Autodesk Inventor part; units mm, degrees
ref_plane "YZ Plane" through (0, 0, 0) normal (1, 0, 0) x (0, 1, 0)
ref_plane "XZ Plane" through (0, 0, 0) normal (0, 1, 0) x (-1, 0, 0)
ref_plane "XY Plane" through (0, 0, 0) normal (0, 0, 1) x (1, 0, 0)
sketch "Sketch1" plane through (0, 0, 0) normal (0, 0, 1) x (1, 0, 0)
  line L0 (-23, -40) -> (23, -40)
  line L1 (23, -40) -> (23, 40)
  line L2 (23, 40) -> (-23, 40)
  line L3 (-23, 40) -> (-23, -40)
  line L4 (-23, -40) -> (23, 40) construction
  line L5 (23, -40) -> (-23, 40) construction
  line L6 (10, -20) -> (-10, -20)
  line L7 (-10, -20) -> (-10, 20)
  line L8 (-10, 20) -> (10, 20)
  line L9 (10, 20) -> (10, -20)
  line L10 (10, -20) -> (-10, 20) construction
  line L11 (-10, -20) -> (10, 20) construction
  point P0 (0, 0)
  dimension "d154" = 46
  dimension "d155" = 80
  dimension "d172" = 20
  dimension "d181" = 40
extrude "Plate5" add sketch "Sketch1" along normal blind 3 contours L3 L2 L1 L0 | L6 L7 L8 L9
sketch "Sketch9" plane through (0, 0, 3) normal (0, 0, 1) x (1, 0, 0)
  circle A0 centre (16.7705, -33.541) radius 3
  line L0 (16.7705, 33.541) -> (-16.7705, 33.541) construction
  line L1 (-16.7705, 33.541) -> (-16.7705, -33.541) construction
  line L2 (-16.7705, -33.541) -> (16.7705, -33.541) construction
  line L3 (16.7705, -33.541) -> (16.7705, 33.541) construction
  line L4 (16.7705, 33.541) -> (-16.7705, -33.541) construction
  line L5 (-16.7705, 33.541) -> (16.7705, -33.541) construction
  circle A1 centre (-16.7705, -33.541) radius 3
  circle A2 centre (16.7705, 33.541) radius 3
  circle A3 centre (-16.7705, 33.541) radius 3
  circle A4 centre (0, 0) radius 37.5 construction
  line L6 (23, -40) -> (-23, -40) construction
  line L7 (23, 40) -> (23, -40) construction
  line L8 (-23, 40) -> (23, 40) construction
  line L9 (-23, -40) -> (-23, 40) construction
  circle A5 centre (0, 0) radius 22.3607 construction
  line L10 (10, 20) -> (-10, -20) construction
  dimension "d180" = 75
  dimension "d182" = 15.1393
  dimension "d174" = 6
  dimension "d183" = 33.541
extrude "Cut2" cut sketch "Sketch9" against normal blind 3
fillet "Corner Round1" radius 6 4 edges at (23, 40, 1.5) (-23, 40, 1.5) (-23, -40, 1.5) (23, -40, 1.5)
feature "Corner Round2" [suppressed]
properties part number "ANP 1434 BOTTOM FDS support flange" material "Stainless Steel"
The listing builds one solid part. Answer for the finished solid, in the listing's coordinates (mm). Coordinates: 2 decimals unless noted, no trailing zeros. Write each loop counter-clockwise with the first axis right and the second up, starting at its lowest first coordinate (ties: lowest second). Pieces come first, ordered by that corner, then holes.
Q1. Given P1, Ø5.5, axis at x = -16.77, y = 33.54, coming from the -Z side, flat-ended and moving along its own axis, determine where the tip first touches the part or whether it passes through.
Returned:
P1: passes through
Q2. The mould has two halves that part along Y. Classify faces 1 (the cylindrical face through (-21.289, -38.196, 1.521)), 2 (the cylindrical face through (-15.16, 36.07, 1.52)), 3 (the flat face through (23, 0, 1)), 4 (the cylindrical face through (-21.196, 38.289, 1.521)): released by +Y, released by -Y, zero draft, split by the parting line, or undercut.
Returned:
face 1: released by -Y
face 2: undercut
face 3: zero draft
face 4: released by +Y
Q3. Section A-A, the plane x = -15 is taken. Write down the section's boundary in (y, z), then the cut area to 3 significant figures.
Returned:
outline: (-40, 0) - (-35.96, 0) - (-35.96, 3) - (-40, 3) - close; (-31.12, 0) - (31.12, 0) - (31.12, 3) - (-31.12, 3) - close; (35.96, 0) - (40, 0) - (40, 3) - (35.96, 3) - close
area: 211 mm2
Q4. Find the intervals of material crossed by line 1 along X through (y, z) = (35, 0.75); line 2 along X through (y, z) = (-32, 1.15); line 3 along Y through (x, z) = (14.5, 2.85), in increasing order.
Returned:
line 1: x = -22.92 to -19.39, -14.15 to 14.15, 19.39 to 22.92
line 2: x = -23 to -19.34, -14.2 to 14.2, 19.34 to 23
line 3: y = -40 to -35.5, -31.58 to 31.58, 35.5 to 40
Q5. Section B-B, the plane z = 0.7 is taken. Write down the section's boundary in (x, y), then the cut area to 3 significant figures.
Returned:
outline: (-23, -34) arc R6 ccw to (-17, -40) - (17, -40) arc R6 ccw to (23, -34) - (23, 34) arc R6 ccw to (17, 40) - (-17, 40) arc R6 ccw to (-23, 34) - close; hole circle Ø6 at (-16.77, -33.54); hole circle Ø6 at (-16.77, 33.54); hole circle Ø6 at (16.77, -33.54); hole circle Ø6 at (16.77, 33.54)
area: 3,540 mm2
